Can you work these out from the model? Positions are in its coordinate system, mm. Face numbers are marked on the shaded views. Round coordinates to 2 decimals unless told otherwise and drop trailing zeros. Order: outer loops, then holes, each group sorted by start corner. A loop starts at its lowest first (then second) coordinate and runs counter-clockwise, first axis right, second up. Notation, with made-up numbers: (10, 89.25) -> (33, 89.25) arc R28 cw to (33, 109.25) -> close; hole circle Ø7 at (-35, 52). An arc over 180 degrees is marked (long way). One line per item, written item: value.
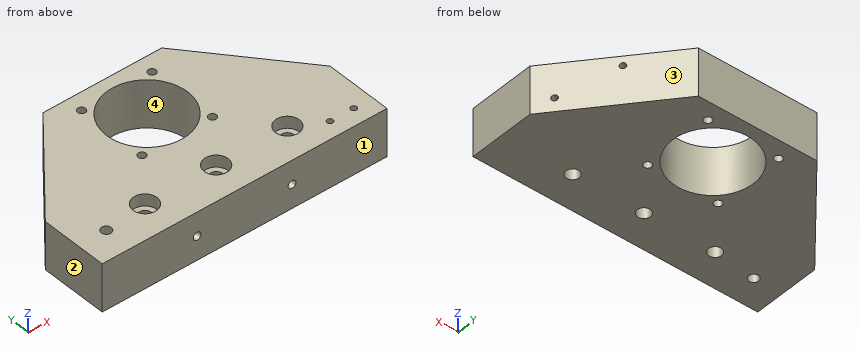
```python
from build123d import *

# Parameters (mm, degrees)
BOSS_EXTRUDE1_DEPTH            = 20
CBORE_FOR_M5_SHCS1_D           = 5.5
CBORE_FOR_M5_SHCS1_CBORE_D     = 10
CBORE_FOR_M5_SHCS1_CBORE_DEPTH = 5
SKETCH4_R                      = 17
CUT_EXTRUDE1_DEPTH             = 95.339811321
M4_TAPPED_HOLE1_D              = 3.3
M4_TAPPED_HOLE2_D              = 3.3
M4_TAPPED_HOLE2_DEPTH          = 15
M4_TAPPED_HOLE2_TIP            = 0.991420021
M3_TAPPED_HOLE1_D              = 2.5
M3_TAPPED_HOLE1_DEPTH          = 7.5
M3_TAPPED_HOLE1_TIP            = 0.751075774
M3_TAPPED_HOLE2_D              = 2.5
M3_TAPPED_HOLE2_DEPTH          = 11.5
M3_TAPPED_HOLE2_TIP            = 0.751075774
M5_TAPPED_HOLE1_D              = 4.2


with BuildPart() as part:
    # Sketch1 → Boss-Extrude1 (new body)
    with BuildSketch(Plane.XY):
        Polygon((60, 0), (-60, 0), (-60, 28), (-25, 70), (25, 70), (60, 28), align=None)
    extrude(amount=BOSS_EXTRUDE1_DEPTH)

    # CBORE for M5 SHCS1 (through all)
    with Locations(Plane(origin=(-30, 14, 20), x_dir=(1, 0, 0), z_dir=(0, 0, 1))):
        with Locations((0, 0), (30, 0), (60, 0)):
            CounterBoreHole(CBORE_FOR_M5_SHCS1_D / 2, CBORE_FOR_M5_SHCS1_CBORE_D / 2, CBORE_FOR_M5_SHCS1_CBORE_DEPTH)

    # Sketch4 → Cut-Extrude1 (cut, through all)
    with BuildSketch(Plane.XY.offset(20)):
        with Locations((0, 48)):
            Circle(SKETCH4_R)
    extrude(amount=-CUT_EXTRUDE1_DEPTH, mode=Mode.SUBTRACT)

    # M4 Tapped Hole1 (through all)
    with Locations(Plane(origin=(-14.849242405, 62.849242405, 20), x_dir=(1, 0, 0), z_dir=(0, 0, 1))):
        with Locations((0, 0), (29.69848481, 0), (29.69848481, -29.69848481), (0, -29.69848481)):
            Hole(M4_TAPPED_HOLE1_D / 2)

    # M4 Tapped Hole2
    with Locations(Plane(origin=(0, 0, 0), x_dir=(-1, 0, 0), z_dir=(0, -1, 0))):
        with Locations((20, -10), (-20, -10)):
            Hole(M4_TAPPED_HOLE2_D / 2, depth=M4_TAPPED_HOLE2_DEPTH)
            with Locations((0, 0, -(M4_TAPPED_HOLE2_DEPTH + M4_TAPPED_HOLE2_TIP / 2))):  # 118° drill point
                Cone(0, M4_TAPPED_HOLE2_D / 2, M4_TAPPED_HOLE2_TIP, mode=Mode.SUBTRACT)

    # M3 Tapped Hole1
    with Locations(Plane(origin=(42, 7, 20), x_dir=(1, 0, 0), z_dir=(0, 0, 1))):
        with Locations((0, 0), (10, 0)):
            Hole(M3_TAPPED_HOLE1_D / 2, depth=M3_TAPPED_HOLE1_DEPTH)
            with Locations((0, 0, -(M3_TAPPED_HOLE1_DEPTH + M3_TAPPED_HOLE1_TIP / 2))):  # 118° drill point
                Cone(0, M3_TAPPED_HOLE1_D / 2, M3_TAPPED_HOLE1_TIP, mode=Mode.SUBTRACT)

    # M3 Tapped Hole2
    with Locations(Plane(origin=(49.180327869, 40.983606557, 0), x_dir=(0, 0, -1), z_dir=(0.7682212795973757, 0.6401843996644799, 0))):
        with Locations((-16, 13.299131849), (-5.7, -8.900868151)):
            Hole(M3_TAPPED_HOLE2_D / 2, depth=M3_TAPPED_HOLE2_DEPTH)
            with Locations((0, 0, -(M3_TAPPED_HOLE2_DEPTH + M3_TAPPED_HOLE2_TIP / 2))):  # 118° drill point
                Cone(0, M3_TAPPED_HOLE2_D / 2, M3_TAPPED_HOLE2_TIP, mode=Mode.SUBTRACT)

    # M5 Tapped Hole1 (through all)
    with Locations(Plane.XY.offset(20)):
        with Locations((-48, 12)):
            Hole(M5_TAPPED_HOLE1_D / 2)


solid = part.part
```
Q1. I want a section at C-C on x = 0. List the corners of the cut face in (y, z) for me, plus the area to 4 significant figures.
Answers below:
outline: (0, 0) -> (11.25, 0) -> (11.25, 15) -> (9, 15) -> (9, 20) -> (0, 20) -> close; (16.75, 0) -> (31, 0) -> (31, 20) -> (19, 20) -> (19, 15) -> (16.75, 15) -> close; (65, 0) -> (70, 0) -> (70, 20) -> (65, 20) -> close
area: 587.5 mm^2
Q2. I want a section at A-A on x = -48. List the corners of the cut face in (y, z) for me, plus the area to 3 significant figures.
Answers below:
outline: (0, 0) -> (9.9, 0) -> (9.9, 20) -> (0, 20) -> close; (14.1, 0) -> (42.4, 0) -> (42.4, 20) -> (14.1, 20) -> close
area: 764 mm^2
Q3. I want a section at B-B on y = 36.5. List the corners of the cut face in (x, z) for me.
Answers below:
outline: (-52.92, 0) -> (-12.52, 0) -> (-12.52, 20) -> (-52.92, 20) -> close; (12.52, 0) -> (52.92, 0) -> (52.92, 20) -> (12.52, 20) -> close
Q4. I want a section at D-D on z = 2. Give the number of separate pieces and of enclosed holes in the cut face, plus the area to 3 significant figures.
Answers below:
separate pieces: 1
enclosed holes: 9
area: 5,900 mm^2
Q5. Please list where these lines run through material, in increasing order: line 1 along Y through (x, z) = (0, 9.5); line 2 along Z through (x, y) = (20, 10.25); line 3 along Y through (x, z) = (-14.5, 2).
Answers below:
line 1: 0 to 11.25, 16.75 to 31, 65 to 70
line 2: 0 to 8.35, 11.65 to 20
line 3: 0 to 31.54, 34.76 to 39.13, 56.87 to 61.24, 64.46 to 70
Q6. Will these pins go through, and if not, where does the flat tip stop? pin 1 Ø3.5 at (x, y) = (-48, 12) entering from +Z (3 decimals); pin 2 Ø8 at (x, y) = (-30, 14) entering from +Z; pin 3 Ø1.5 at (y, z) = (41, 8) entering from -X; pin 4 Ø1 at (x, z) = (-44.5, 11.5) entering from +Y.
Answers below:
pin 1: through
pin 2: z = 15
pin 3: x = -49.79
pin 4: y = 47.2
Q7. We'd pull the mould along X, two halves only. Please class the marked faces 1, 2, 3 and 4: released by +X, released by -X, zero draft, split by the parting line, or undercut.
Answers below:
face 1: zero draft
face 2: released by -X
face 3: released by +X
face 4: undercut
